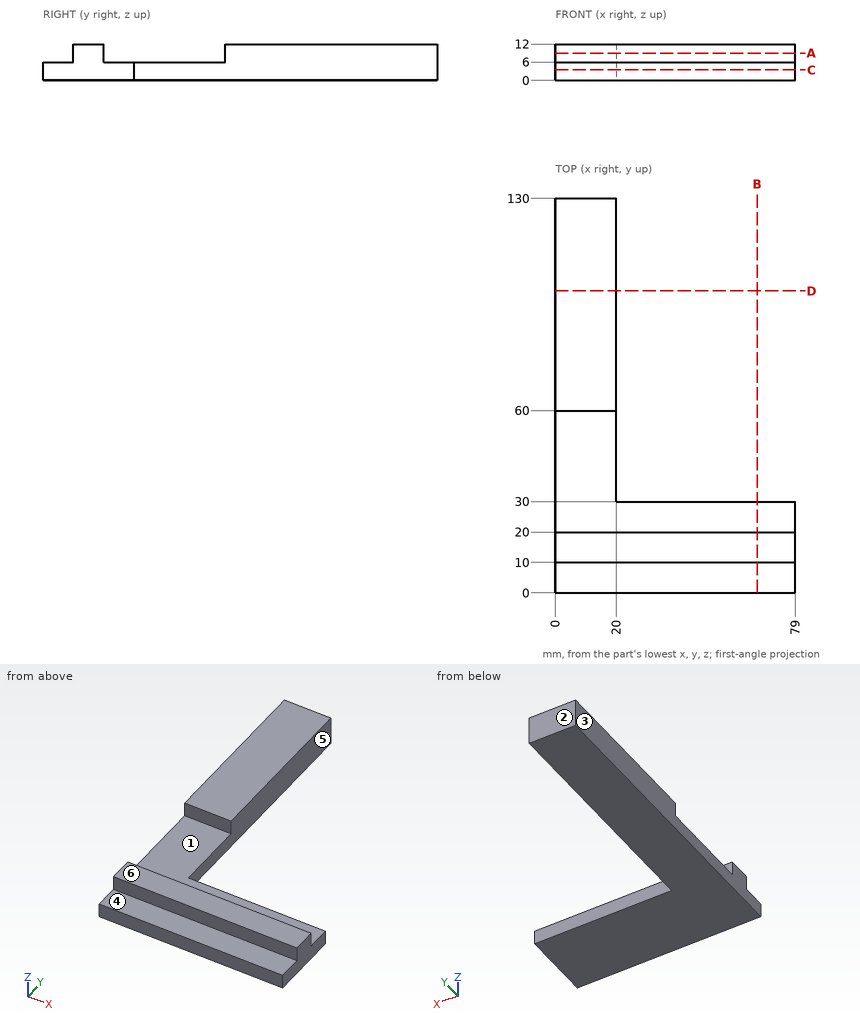
Check sheet for the drawn part. Datum: minimum x, y, z corner. Units: mm. A direction names the side the tool comes from. Coordinates: 2 decimals unless noted, no trailing zeros. Loops run counter-clockwise (first coordinate to the right, second up) from the corner with the lowest first, then second, coordinate; pieces in that order, holes last. Notation, with made-up numbers: (86.25, -25) -> (138.25, -25) arc R31 cw to (138.25, 3) -> close; hole circle Ø7 at (74, 3.25). An arc over 180 degrees is marked (long way). Answer as CSV lines item,"result".
1) Depth check by flat-ended pin: pin 1 (1.8 mm diameter, centred on x = 8, z = 7.5, fed in from -Y); pin 2 (1.8 mm diameter, centred on x = 28.5, z = 9, fed in from +Y); pin 3 (3 mm diameter, centred on x = 51, z = 3.5, fed in from +Y). Enter the tip coordinate at first touch or a pass-through.
Found:
pin 1,"stops at y = 10"
pin 2,"stops at y = 20"
pin 3,"stops at y = 30"
2) Cross-section at D-D, the plane y = 99.5. Record the cut outline in (x, z).
Found:
outline,"(0, 0) -> (20, 0) -> (20, 12) -> (0, 12) -> close"
3) Cross-section at A-A, the plane z = 9. Record the cut outline in (x, y), then the cut area to 3 significant figures.
Found:
outline,"(0, 10) -> (79, 10) -> (79, 20) -> (0, 20) -> close; (0, 60) -> (20, 60) -> (20, 130) -> (0, 130) -> close"
area,"2,190 mm2"
4) Cross-section at B-B, the plane x = 66.5. Record the cut outline in (y, z), then the cut area to 3 significant figures.
Found:
outline,"(0, 0) -> (30, 0) -> (30, 6) -> (20, 6) -> (20, 12) -> (10, 12) -> (10, 6) -> (0, 6) -> close"
area,"240 mm2"
5) Thickness scan on L1, parallel to X at y = 106, z = 6.5; L2, parallel to Z at x = 37.5, y = 24; L3, parallel to Y at x = 26, z = 9.5. Record the ranges inside material, lowest first. Write a range as from..to.
Found:
L1,"x = 0..20"
L2,"z = 0..6"
L3,"y = 10..20"
6) Tool access check on the marked faces 4, 5 and 6. Record the directions out of +Z, -Z, +X, -X, +Y, -Y that give a thin tool (end or side, any length) a straight path to the whole face; none if there is none.
Found:
face 4,"+Z, +X, -X, -Y"
face 5,"+Z, -Z, +X, +Y"
face 6,"+Z, +X, -X, +Y, -Y"
7) Release check for a two-part mould opening along Y. For the marked faces 1, 2 and 3 record: +Y half, -Y half, draft (parallel to the pull), parting line (faces both ways), or undercut.
Found:
face 1,"undercut"
face 2,"+Y half"
face 3,"draft"
8) Cross-section at C-C, the plane z = 3.5. Record the cut outline in (x, y).
Found:
outline,"(0, 0) -> (79, 0) -> (79, 30) -> (20, 30) -> (20, 130) -> (0, 130) -> close"
